Here's how the part is built. I have some questions about the finished solid (model axes, mm). Face numbers are marked on the shaded views. Coordinates: 2 decimals unless noted, no trailing zeros. Write each loop counter-clockwise with the first axis right and the second up, starting at its lowest first coordinate (ties: lowest second). Pieces come first, ordered by that corner, then holes.
(1) For pin 1 Ø5 at (x, z) = (-19, 0) entering from +Y; pin 2 Ø3.5 at (x, y) = (0, 8.5) entering from +Z; pin 3 Ø1.6 at (y, z) = (7.5, -35) entering from +X; pin 4 Ø12 at (x, z) = (-13, 1.5) entering from -Y, each with a flat end and sliding along its axis, tell me the tip position at first contact or that it passes through.
(2) Imagine slicing it at D-D, the plane x = -3. List the corners of the cut face in (y, z) for me, plus the area to 3 significant figures.
(3) Thinking about a two-plate mould opening in Z: for the marked faces 1 and 2, which applies, released by +Z, released by -Z, zero draft, split by the parting line, or undercut?
(4) Imagine slicing it at A-A, the plane x = 19. List the corners of the cut face in (y, z) for me, plus the area to 3 significant figures.
(5) Imagine slicing it at C-C, the plane z = -44. List the corners of the cut face in (x, y) for me.
(6) Please list where these lines run through material, in increasing order: probe 1 along X at (y, z) = (0.55, -44); probe 2 along Z at (x, y) = (-19, 0.9); probe 3 along Z at (x, y) = (0.5, 6.75).
(7) Imagine slicing it at B-B, the plane z = -16. List the corners of the cut face in (x, y) for me.
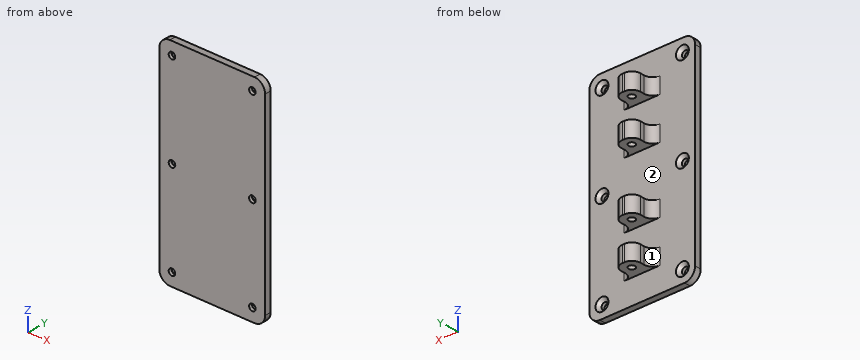
Autodesk Inventor part; units mm, degrees
ref_plane "YZ Plane" through (0, 0, 0) normal (1, 0, 0) x (0, 1, 0)
ref_plane "XZ Plane" through (0, 0, 0) normal (0, 1, 0) x (-1, 0, 0)
ref_plane "XY Plane" through (0, 0, 0) normal (0, 0, 1) x (1, 0, 0)
sketch "Sketch1" plane through (0, 0, 0) normal (0, 1, 0) x (-1, 0, 0)
  line L0 (25, 50) -> (-25, 50)
  line L1 (-25, 50) -> (-25, -50)
  line L2 (-25, -50) -> (25, -50)
  line L3 (25, -50) -> (25, 50)
  point P0 (0, 0)
  dimension "d0" = 100
  dimension "d1" = 50
  dimension "d2" = 25
  dimension "d3" = 50
extrude "Extrusion1" add sketch "Sketch1" along normal blind 3
sketch "Sketch2" plane through (0, 3, 0) normal (0, 1, 0) x (1, 0, 0)
  line L0 (-4.5, -30.5) -> (4.5, -30.5)
  line L1 (4.5, -30.5) -> (4.5, -19.5)
  line L2 (4.5, -19.5) -> (-4.5, -19.5)
  line L3 (-4.5, -19.5) -> (-4.5, -30.5)
  line L4 (-4.5, -19.5) -> (-4.5, -19)
  line L5 (-4.5, -19) -> (4.5, -19)
  line L6 (4.5, -19) -> (4.5, -19.5)
  line L7 (-4.5, -19) -> (-4.5, -11.5)
  line L8 (-4.5, -11.5) -> (4.5, -11.5)
  line L9 (4.5, -11.5) -> (4.5, -19)
  line L10 (-4.5, -30.5) -> (-4.5, -31)
  line L11 (-4.5, -31) -> (4.5, -31)
  line L12 (4.5, -31) -> (4.5, -30.5)
  line L13 (-4.5, -31) -> (-4.5, -38.5)
  line L14 (-4.5, -38.5) -> (4.5, -38.5)
  line L15 (4.5, -38.5) -> (4.5, -31)
  line L16 (-25, -50) -> (25, -50)
  line L17 (31.6742, 0) -> (-41.419, 0)
  line L18 (-4.5, 30.5) -> (4.5, 30.5)
  line L19 (4.5, 30.5) -> (4.5, 19.5)
  line L20 (4.5, 19.5) -> (-4.5, 19.5)
  line L21 (-4.5, 19.5) -> (-4.5, 30.5)
  line L22 (-4.5, 19.5) -> (-4.5, 19)
  line L23 (-4.5, 19) -> (4.5, 19)
  line L24 (4.5, 19) -> (4.5, 19.5)
  line L25 (-4.5, 19) -> (-4.5, 11.5)
  line L26 (-4.5, 11.5) -> (4.5, 11.5)
  line L27 (4.5, 11.5) -> (4.5, 19)
  line L28 (-4.5, 30.5) -> (-4.5, 31)
  line L29 (-4.5, 31) -> (4.5, 31)
  line L30 (4.5, 31) -> (4.5, 30.5)
  line L31 (-4.5, 31) -> (-4.5, 38.5)
  line L32 (-4.5, 38.5) -> (4.5, 38.5)
  line L33 (4.5, 38.5) -> (4.5, 31)
  line L34 (-25, 50) -> (-25, -50)
  line L35 (25, -50) -> (25, 50)
  line L36 (25, 50) -> (-25, 50)
  point P0 (0, 0)
  point P1 (-19, -44)
  point P2 (-19, 0)
  point P3 (-19, 44)
  point P4 (19, -44)
  point P5 (19, 0)
  point P6 (19, 44)
  dimension "d6" = 9
  dimension "d7" = 11
  dimension "d8" = 4.5
  dimension "d9" = 0.5
  dimension "d10" = 0.5
  dimension "d11" = 27
  dimension "d12" = 7.5
  dimension "d14" = 11.5
  dimension "d27" = 6
  dimension "d28" = 6
  dimension "d29" = 6
  dimension "d30" = 6
  dimension "d31" = 50
  dimension "d43" = 39
extrude "Extrusion2" add sketch "Sketch2" along normal blind 10 contours L11 L15 L14 L13 | L7 L8 L9 L5 | L31 L32 L33 L29 | L23 L27 L26 L25
sketch "Sketch3" plane through (-4.5, 3, 38.5) normal (0, 0, 1) x (1, 0, 0)
  line L0 (9, 0) -> (0, 0)
  line L1 (9, 0) -> (9, 10)
  line L2 (0, 10) -> (9, 10)
  line L3 (0, 0) -> (0, 10)
  point P0 (4.5, -3)
  point P1 (4.5, 5.5)
  point P2 (4.5, 10)
  dimension "d17" = 4.5
  dimension "d18" = 4.5
hole "Hole1" at (0, 8.5, 38.5) direction (0, 0, -1) diameter 3.1 end through all
fillet "Fillet1" radius 4 16 edges at (-4.5, 13, 34.75) (4.5, 13, 34.75) (-4.5, 13, 15.25) (4.5, 13, 15.25) (-4.5, 13, -15.25) (4.5, 13, -15.25) (-4.5, 13, -34.75) (4.5, 13, -34.75) (-4.5, 3, -34.75) (-4.5, 3, -15.25) (-4.5, 3, 15.25) (-4.5, 3, 34.75) (4.5, 3, 34.75) (4.5, 3, 15.25) (4.5, 3, -15.25) (4.5, 3, -34.75)
hole "Hole2" at (-19, 3, 44) at (-19, 3, 0) at (-19, 3, -44) at (19, 3, 44) at (19, 3, 0) at (19, 3, -44) direction (0, -1, 0) diameter 3.1 end through all
chamfer "Chamfer1" distance 1.5 angle 45 6 edges at (19, 3, -45.55) (19, 3, -1.55) (-19, 3, -45.55) (19, 3, 42.45) (-19, 3, -1.55) (-19, 3, 42.45)
fillet "Fillet2" radius 5 4 edges at (25, 1.5, 50) (-25, 1.5, 50) (-25, 1.5, -50) (25, 1.5, -50)
equation "\"d10\" = d9"
equation "\"d12\" = -0.5 * d10 - 0.5 * d7 + 0.5 * d11 - 0.5 * d9"
properties part number "3DP_PLA_Stand_Leg_Mount"
Recorded:
1. pin 1: stops at y = 2.45
1. pin 2: stops at z = 38.5
1. pin 3: stops at x = 4.51
1. pin 4: stops at y = 0
2. outline: (0, -50) - (3, -50) - (3, -38.5) - (12.12, -38.5) - (12.12, -31) - (3, -31) - (3, -19) - (12.12, -19) - (12.12, -11.5) - (3, -11.5) - (3, 11.5) - (12.12, 11.5) - (12.12, 19) - (3, 19) - (3, 31) - (12.12, 31) - (12.12, 38.5) - (3, 38.5) - (3, 50) - (0, 50) - close
2. area: 574 mm2
3. face 1: zero draft
3. face 2: undercut
4. outline: (0, -50) - (3, -50) - (3, -47.05) - (1.5, -45.55) - (0, -45.55) - close; (0, -42.45) - (1.5, -42.45) - (3, -40.95) - (3, -3.05) - (1.5, -1.55) - (0, -1.55) - close; (0, 1.55) - (1.5, 1.55) - (3, 3.05) - (3, 40.95) - (1.5, 42.45) - (0, 42.45) - close; (0, 45.55) - (1.5, 45.55) - (3, 47.05) - (3, 50) - (0, 50) - close
4. area: 265 mm2
5. outline: (-25, 0) - (-20.55, 0) - (-20.55, 1.5) - (-22.05, 3) - (-25, 3) - close; (-17.45, 0) - (17.45, 0) - (17.45, 1.5) - (15.95, 3) - (-15.95, 3) - (-17.45, 1.5) - close; (20.55, 0) - (25, 0) - (25, 3) - (22.05, 3) - (20.55, 1.5) - close
6. probe 1: x = -25 to -20.55, -17.45 to 17.45, 20.55 to 25
6. probe 2: z = -50 to -45.55, -42.45 to -1.55, 1.55 to 42.45, 45.55 to 50
6. probe 3: z = -38.5 to -31, -19 to -11.5, 11.5 to 19, 31 to 38.5
7. outline: (-25, 0) - (25, 0) - (25, 3) - (8.5, 3) arc R4 cw to (4.5, 7) - (4.5, 9) arc R4 ccw to (0.5, 13) - (-0.5, 13) arc R4 ccw to (-4.5, 9) - (-4.5, 7) arc R4 cw to (-8.5, 3) - (-25, 3) - close; hole circle Ø3.1 at (0, 8.5)
